Verification items for this drawing (mm, ordinates from the low corner). A direction names the side the tool comes from. Round coordinates to 2 decimals unless told otherwise and drop trailing zeros. Loops run counter-clockwise (first coordinate to the right, second up) from the corner with the lowest first, then second, coordinate; pieces in that order, holes last. Notation, with made-up numbers: (-9.75, -5.5) - (27.25, -5.5) arc R22 cw to (27.25, 23.5) - close; hole circle Ø3 at (-19.5, 53.25). An arc over 180 degrees is marked (long way). Write item = value, one per line.
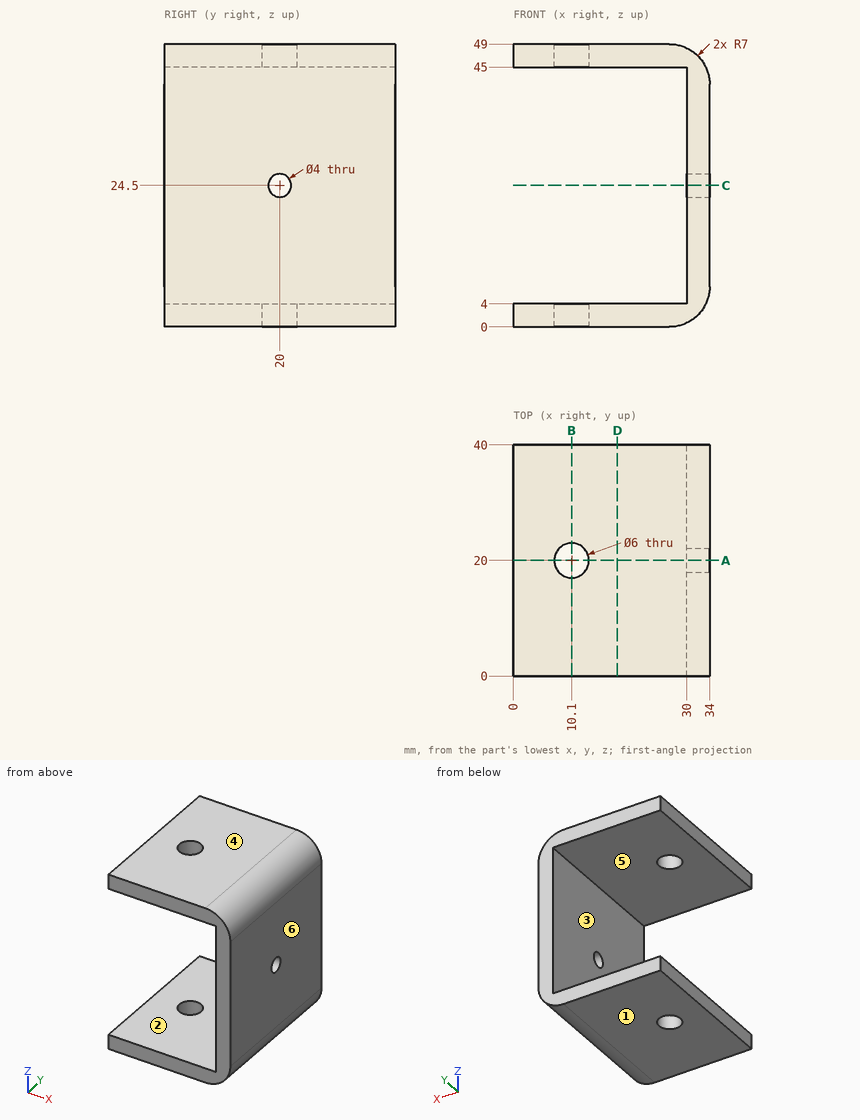
(1) Section check A-A (y = 20). Enter the section's corners in (x, z), then the cut area to 3 significant figures.
Answers follow:
outline = (0, 0) - (7.1, 0) - (7.1, 4) - (0, 4) - close; (0, 45) - (7.1, 45) - (7.1, 49) - (0, 49) - close; (13.1, 0) - (27, 0) arc R7 ccw to (34, 7) - (34, 22.5) - (30, 22.5) - (30, 4) - (13.1, 4) - close; (13.1, 45) - (30, 45) - (30, 26.5) - (34, 26.5) - (34, 42) arc R7 ccw to (27, 49) - (13.1, 49) - close
area = 351 mm²
(2) Mould release check, pull along Z, two halves, no side actions. Record for the marked faces 3, 4, 5 and 6: pulls with the +Z half, pulls with the -Z half, needs draft (parallel to the pull), parting line crosses it, or undercut.
Answers follow:
face_3 = undercut
face_4 = pulls with the +Z half
face_5 = undercut
face_6 = needs draft
(3) Scan lines: L1, parallel to Z at x = 13, y = 24; L2, parallel to X at y = 17, z = 30.5; L3, parallel to Z at x = 32.2, y = 20. Record each from-to range of solid material in increasing order. Write a range as [from, to].
Answers follow:
L1 = [0, 4], [45, 49]
L2 = [30, 34]
L3 = [2.31, 22.5], [26.5, 46.69]
(4) Section check D-D (x = 18). Enter the section's corners in (y, z).
Answers follow:
outline = (0, 0) - (40, 0) - (40, 4) - (0, 4) - close; (0, 45) - (40, 45) - (40, 49) - (0, 49) - close
(5) Section check B-B (x = 10.1). Enter the section's corners in (y, z), then the cut area to 3 significant figures.
Answers follow:
outline = (0, 0) - (17, 0) - (17, 4) - (0, 4) - close; (0, 45) - (17, 45) - (17, 49) - (0, 49) - close; (23, 0) - (40, 0) - (40, 4) - (23, 4) - close; (23, 45) - (40, 45) - (40, 49) - (23, 49) - close
area = 272 mm²
(6) Section check C-C (z = 24.5). Enter the section's corners in (x, y).
Answers follow:
outline = (30, 0) - (34, 0) - (34, 18) - (30, 18) - close; (30, 22) - (34, 22) - (34, 40) - (30, 40) - close
(7) Gauge pin test, flat end, axial feed: pin 1 (4.5 mm diameter, centred on y = 20, z = 24.5, fed in from -X). Record the tip position at first contact, or that the pin passes through.
Answers follow:
pin_1 = 30
(8) Set-up check for the marked faces 1 and 2: record each of +Z, -Z, +X, -X, +Y, -Y from which the full face is reachable in a straight line by a thin tool's end or side.
Answers follow:
face_1 = -Z, +X, -X, +Y, -Y
face_2 = -X, +Y, -Y
